Could you check a few things on this model? Use its own coordinates, in mm. Coordinates: 2 decimals unless noted, no trailing zeros. Loops run counter-clockwise (first coordinate to the right, second up) from the corner with the lowest first, then second, coordinate; pieces in that order, holes last. Notation, with made-up numbers: M -35,-8 L -28,-8 A13 ccw -28,11 Z; hole C -2.75,-24 d10. An arc over 180 degrees is marked long. Write each question's results on one line, items separated by ' | '.
```python
from build123d import *

# Parameters (mm, degrees)
SKETCH1_W           = 50.8
SKETCH1_H           = 57.15
BOSS_EXTRUDE1_DEPTH = 6.35
CUT_EXTRUDE1_REACH  = 14.7
SKETCH2_R           = 15.875
FILLET1_R           = 25.4


with BuildPart() as part:
    # Sketch1 → Boss-Extrude1 (new body, symmetric)
    with BuildSketch(Plane(origin=(0, 0, 0), x_dir=(0, 0, -1), z_dir=(1, 0, 0))):
        Rectangle(SKETCH1_W, SKETCH1_H)
    extrude(amount=BOSS_EXTRUDE1_DEPTH, both=True)

    # Sketch2 → Cut-Extrude1 (cut, up to next)
    with BuildSketch(Plane(origin=(6.35, 0, 0), x_dir=(0, 0, -1), z_dir=(1, 0, 0)), mode=Mode.PRIVATE) as cut_extrude1_sk1:
        with Locations((0, 3.175)):
            Circle(SKETCH2_R)
    cut_extrude1_tool1 = extrude(cut_extrude1_sk1.sketch, amount=-CUT_EXTRUDE1_REACH, mode=Mode.PRIVATE) & part.part
    add(cut_extrude1_tool1.solids().sort_by_distance((6.35, 3.175, 0))[0], mode=Mode.SUBTRACT)

    # Fillet1
    fillet1_edges = [part.edges().sort_by_distance(p)[0] for p in [
        (0, 28.575, -25.4),
    ]]
    fillet(fillet1_edges, radius=FILLET1_R)


solid = part.part
```
(1) If we mould it in two halves opening along Y, with no side actions, what happens to faces 1 (the cylindrical face through (-0.089, 21.332, -17.762)), 2 (the flat face through (6.35, -12, 6)), 3 (the cylindrical face through (0.089, 18.915, 2.067)), 4 (the flat face through (0, -28.575, 0))? For each: released by +Y, released by -Y, zero draft, split by the parting line, or undercut.
Reported:
face 1: released by +Y | face 2: zero draft | face 3: undercut | face 4: released by -Y
(2) Imagine slicing it at B-B, the plane y = -2. List the corners of the cut face in (x, z) for me, and give its area (3 significant figures).
Reported:
outline: M -6.35,-25.4 L 6.35,-25.4 L 6.35,-15.01 L -6.35,-15.01 Z; M -6.35,15.01 L 6.35,15.01 L 6.35,25.4 L -6.35,25.4 Z | area: 264 mm2
(3) Imagine slicing it at D-D, the plane y = 20. List the corners of the cut face in (x, z) for me.
Reported:
outline: M -6.35,-19.03 L 6.35,-19.03 L 6.35,25.4 L -6.35,25.4 Z
(4) Will these pins go through, and if not, where does the flat tip stop? P1, Ø5, axis at x = -1.5, z = -9, coming from the +Y side; P2, Ø3, axis at x = -0.5, z = -20, coming from the +Y side.
Reported:
P1: stops at y = 27.73 | P2: stops at y = 20.58
(5) Imagine slicing it at C-C, the plane x = 2. List the corners of the cut face in (y, z) for me (3 decimals).
Reported:
outline: M -28.575,-25.4 L 3.175,-25.4 A25.4 ccw 28.575,0 L 28.575,25.4 L -28.575,25.4 Z; hole C 3.175,0 d31.75
(6) Please list where these lines run through material, in increasing order: probe 1 along Y at (x, z) = (2.75, 0) (3 decimals); probe 2 along Z at (x, y) = (3.5, 3); probe 3 along Y at (x, z) = (0.5, -13) (3 decimals). Write a range as from..to.
Reported:
probe 1: y = -28.575..-12.7, 19.05..28.575 | probe 2: z = -25.4..-15.87, 15.87..25.4 | probe 3: y = -28.575..-5.936, 12.286..24.996
(7) Imagine slicing it at A-A, the plane z = -4. List the corners of the cut face in (x, y) for me (3 decimals).
Reported:
outline: M -6.35,-28.575 L 6.35,-28.575 L 6.35,-12.188 L -6.35,-12.188 Z; M -6.35,18.538 L 6.35,18.538 L 6.35,28.258 L -6.35,28.258 Z
